For this review, use the dimensioned drawing (mm, ordinates from the lowest corner) and the shaded views. A direction names the side the tool comes from. Coordinates: 2 decimals unless noted, no trailing zeros. Loops run counter-clockwise (first coordinate to the right, second up) from the corner with the lowest first, then second, coordinate; pieces in that order, holes last.
1. Take a section at A-A, the plane z = 65. State the section outline as (x, y) points.
2. To check wall thickness, follow probe 1 along X at (y, z) = (17.5, 65); probe 2 along Z at (x, y) = (16, 11); probe 3 along Z at (x, y) = (23.5, 28). State the ranges of each line that lie inside material, in increasing order.
3. Machinability: for the marked faces 1, 2 and 3, which of the approach directions +Z, -Z, +X, -X, +Y, -Y give a long, thin tool a straight path to every point of the face, cutting with its end or side? Answer none if there is none.
4. Clearance check with flat-ended pins moving along their axes: P1, Ø4, axis at x = 5, y = 23, coming from the -Z side; P2, Ø10, axis at x = 10, y = 7, coming from the +Z side; P3, Ø3.5, axis at x = 18, y = 4, coming from the +Z side. State where each tip first meets the part, or that it passes through.
5. Take a section at C-C, the plane z = 29. State the section outline as (x, y) points.
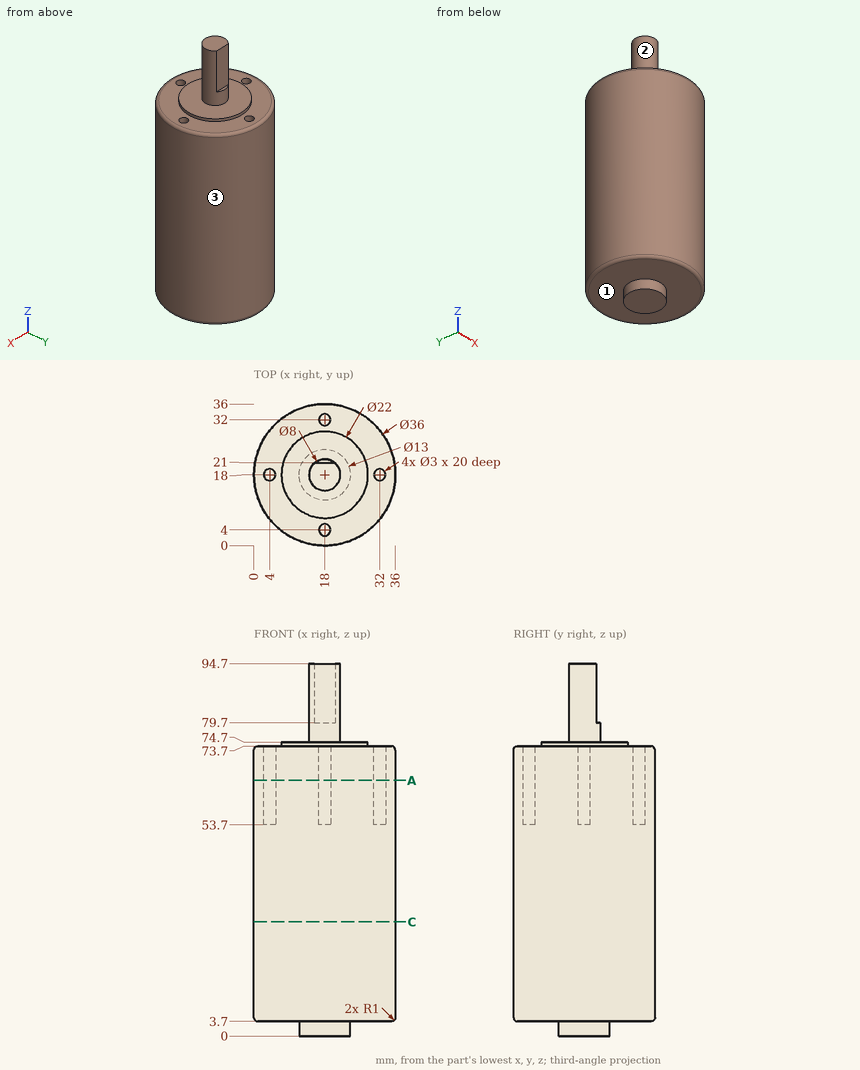
Results list:
1. outline: circle Ø36 at (18, 18); hole circle Ø3 at (4, 18); hole circle Ø3 at (18, 4); hole circle Ø3 at (18, 32); hole circle Ø3 at (32, 18)
2. probe 1: x = 0.01 to 2.59, 5.41 to 30.59, 33.41 to 35.99
2. probe 2: z = 3.7 to 74.7
2. probe 3: z = 3.7 to 73.7
3. face 1: -Z
3. face 2: +Z
3. face 3: +Z, -Z
4. P1: stops at z = 3.7
4. P2: stops at z = 74.7
4. P3: stops at z = 73.7
5. outline: circle Ø36 at (18, 18)
